Input: dimensioned drawing with shaded views. Units: mm. Origin: part minimum x, y, z. A direction names the side the tool comes from. Round coordinates to 2 decimals unless told otherwise and drop trailing zeros. Loops run counter-clockwise (first coordinate to the right, second up) from the corner with the lowest first, then second, coordinate; pieces in that order, holes last. Notation, with made-up numbers: M 54.25,-40 L 58.25,-40 A13 ccw 58.25,-25 Z; hole C 52.5,35 d4. An arc over 180 degrees is marked long. Answer as CSV lines item,"result". Start each with the question number.
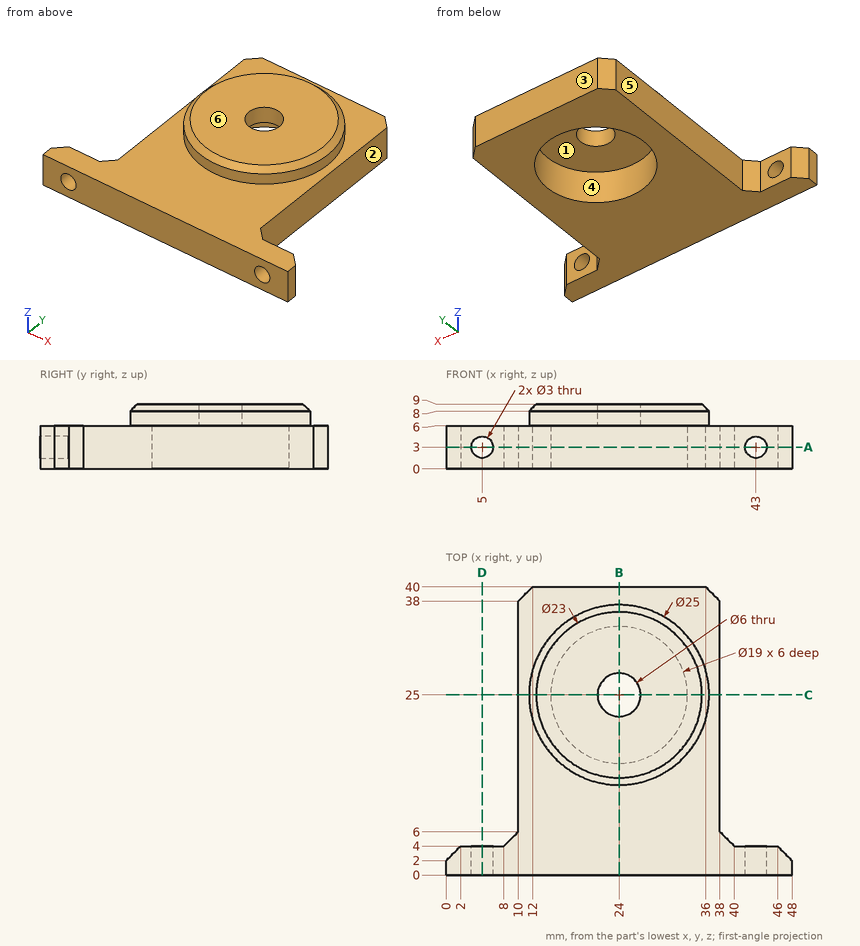
1) Section C-C, the plane y = 25. Return loops of the section in (x, z), and give its area (3 significant figures).
2) Section A-A, the plane z = 3. Return loops of the section in (x, y).
3) Section B-B, the plane x = 24. Return loops of the section in (y, z).
4) Ray query, line 1 along X through (y, z) = (1.8, 3); line 2 along X through (y, z) = (2.2, 3); line 3 along Z through (x, y) = (23.5, 11). Return the intervals inside material, ascending.
5) Contact query for flat-ended pins moving along their axis: pin 1 Ø2 at (x, y) = (37, 4) entering from -Z; pin 2 Ø1.8 at (y, z) = (24, 4) entering from +X; pin 3 Ø5.5 at (x, y) = (24, 25) entering from -Z; pin 4 Ø5.5 at (x, y) = (26.5, 24) entering from -Z. Output: stop coordinate, or through.
6) Access query for the marked faces 5 and 6. Directions: +Z, -Z, +X, -X, +Y, -Y. A direction counts if a zero-diameter tool reaches every point of the face in a straight line with its end or side. Return the directions, or none.
7) Mould query, pull axis X, two halves, no side actions, for the marked faces 1, 2, 3 and 4. Classes: pulls with the +X half, pulls with the -X half, needs draft (parallel to the pull), parting line crosses it, or undercut.
8) Section D-D, the plane x = 5. Return loops of the section in (y, z).
Findings below:
1,outline,"M 10,0 L 14.5,0 L 14.5,6 L 21,6 L 21,9 L 12.5,9 L 11.5,8 L 11.5,6 L 10,6 Z; M 27,6 L 33.5,6 L 33.5,0 L 38,0 L 38,6 L 36.5,6 L 36.5,8 L 35.5,9 L 27,9 Z"
1,area,"110 mm²"
2,outline,"M 0,0 L 3.5,0 L 3.5,4 L 2,4 L 0,2 Z; M 6.5,0 L 41.5,0 L 41.5,4 L 40,4 L 38,6 L 38,38 L 36,40 L 12,40 L 10,38 L 10,6 L 8,4 L 6.5,4 Z; M 44.5,0 L 48,0 L 48,2 L 46,4 L 44.5,4 Z; hole C 24,25 d19"
3,outline,"M 0,0 L 15.5,0 L 15.5,6 L 22,6 L 22,9 L 13.5,9 L 12.5,8 L 12.5,6 L 0,6 Z; M 28,6 L 34.5,6 L 34.5,0 L 40,0 L 40,6 L 37.5,6 L 37.5,8 L 36.5,9 L 28,9 Z"
4,line 1,"0 to 3.5, 6.5 to 41.5, 44.5 to 48"
4,line 2,"0.2 to 3.5, 6.5 to 41.5, 44.5 to 47.8"
4,line 3,"0 to 6"
5,pin 1,"z = 0"
5,pin 2,"x = 38"
5,pin 3,"through"
5,pin 4,"z = 6"
6,face 5,"+Z, -Z, -X, +Y"
6,face 6,"+Z, +X, -X, +Y, -Y"
7,face 1,"undercut"
7,face 2,"pulls with the +X half"
7,face 3,"needs draft"
7,face 4,"undercut"
8,outline,"M 0,0 L 4,0 L 4,1.5 L 0,1.5 Z; M 0,4.5 L 4,4.5 L 4,6 L 0,6 Z"
